Here's how the part is built. I have some questions about the finished solid (model axes, mm). A direction names the side the tool comes from. Coordinates: 2 decimals unless noted, no trailing zeros. Order: outer loops, then holes, each group sorted by start corner. A loop starts at its lowest first (then second) coordinate and runs counter-clockwise, first axis right, second up.
```python
from build123d import *

# Parameters (mm, degrees)
SKETCH1_W           = 30
SKETCH1_H           = 20
SKETCH1_R           = 1.3
BOSS_EXTRUDE1_DEPTH = 5
SKETCH2_W           = 18.5
SKETCH2_H           = 20
BOSS_EXTRUDE2_DEPTH = 70
FILLET1_R           = 1
SKETCH12_W          = 8.5
SKETCH12_H          = 10
CUT_EXTRUDE1_DEPTH  = 81
FILLET2_R           = 1


with BuildPart() as part:
    # Sketch1 → Boss-Extrude1 (new body)
    with BuildSketch(Plane(origin=(0, 0, 0), x_dir=(1, 0, 0), z_dir=(0, 1, 0))):
        Rectangle(SKETCH1_W, SKETCH1_H)
        with Locations((-12, 6)):
            Circle(SKETCH1_R, mode=Mode.SUBTRACT)
        with Locations((12, 6)):
            Circle(SKETCH1_R, mode=Mode.SUBTRACT)
        with Locations((12, -6)):
            Circle(SKETCH1_R, mode=Mode.SUBTRACT)
        with Locations((-12, -6)):
            Circle(SKETCH1_R, mode=Mode.SUBTRACT)
    boss_extrude1 = extrude(amount=BOSS_EXTRUDE1_DEPTH)

    # Sketch2 → Boss-Extrude2 (add)
    with BuildSketch(Plane(origin=(0, 5, 0), x_dir=(1, 0, 0), z_dir=(0, 1, 0))):
        Rectangle(SKETCH2_W, SKETCH2_H)
    extrude(amount=BOSS_EXTRUDE2_DEPTH)

    # Mirror1: Boss-Extrude1 across plane
    add(boss_extrude1.mirror(Plane.ZX.offset(40)))

    # Fillet1
    fillet1_edges = [part.edges().sort_by_distance(p)[0] for p in [
        (-15, 5, 0),
        (-12.125, 5, 10),
        (-12.125, 5, -10),
        (12.125, 5, 10),
        (9.25, 5, 0),
        (9.25, 40, 10),
        (9.25, 40, -10),
        (-9.25, 5, 0),
        (-9.25, 40, -10),
        (-9.25, 40, 10),
        (9.25, 75, 0),
        (-9.25, 75, 0),
        (15, 75, 0),
        (15, 77.5, -10),
        (-12.125, 75, 10),
        (12.125, 75, 10),
        (15, 77.5, 10),
        (-15, 75, 0),
        (-15, 77.5, 10),
        (12.125, 75, -10),
        (-12.125, 75, -10),
        (-15, 77.5, -10),
        (15, 5, 0),
        (15, 2.5, 10),
        (-15, 2.5, 10),
        (-15, 2.5, -10),
        (15, 2.5, -10),
        (12.125, 5, -10),
    ]]
    fillet(fillet1_edges, radius=FILLET1_R)

    # Sketch12 → Cut-Extrude1 (cut, through all)
    with BuildSketch(Plane(origin=(0, 80, 0), x_dir=(1, 0, 0), z_dir=(0, 1, 0))):
        Rectangle(SKETCH12_W, SKETCH12_H)
    extrude(amount=-CUT_EXTRUDE1_DEPTH, mode=Mode.SUBTRACT)

    # Fillet2
    fillet2_edges = [part.edges().sort_by_distance(p)[0] for p in [
        (4.25, 40, 5),
        (-4.25, 40, 5),
        (-4.25, 40, -5),
        (4.25, 40, -5),
    ]]
    fillet(fillet2_edges, radius=FILLET2_R)


solid = part.part
```
Q1. If we section it at B-B on z = -2.5: Write out the boundary of the cut face in (x, y).
Q2. If we section it at C-C on y = 16: Write out the boundary of the cut face in (x, z).
Q3. I need wall thicknesses on L1, parallel to X at y = 4, z = 6; L2, parallel to Z at x = -12, y = 79; L3, parallel to Y at x = 11.5, z = -3.5. Which ranges of each line are inside material? Lowest first, please.
Q4. If we section it at D-D on x = 12: Write out the boundary of the cut face in (y, z).
Q5. We'd pull the mould along Z, two halves only. Please class faces 1 (the flat face through (-12, 5, 0)), 2 (the flat face through (0, 41, 10)), 3 (the cylindrical face through (-11.4, 77.535, 7.153)), 4 (the flat face through (4.25, 41, 0)): pulls with the +Z half, pulls with the -Z half, needs draft (parallel to the pull), parting line crosses it, or undercut.
Q6. If we section it at A-A on x = -2.5: Write out the boundary of the cut face in (y, z).
Q7. Will these pins go through, and if not, where does the flat tip stop? pin 1 (9 mm diameter, centred on y = 41.5, z = -4, fed in from +X); pin 2 (2 mm diameter, centred on y = 52.5, z = -1, fed in from -X).
Q8. For faces 5 (the flat face through (0, 41, -5)), 6 (the flat face through (15, 78, 0)), 7 (the flat face through (12, 75, 0)), 8 (the flat face through (-12, 75, 0)), which set-ups out of +Z, -Z, +X, -X, +Y, -Y let a thin tool reach every point of the face, with its end or its side?
Reply:
1. outline: (-15, 0) - (-4.25, 0) - (-4.25, 80) - (-15, 80) - (-15, 76) arc R1 ccw to (-14, 75) - (-10.25, 75) arc R1 cw to (-9.25, 74) - (-9.25, 6) arc R1 cw to (-10.25, 5) - (-14, 5) arc R1 ccw to (-15, 4) - close; (4.25, 0) - (15, 0) - (15, 4) arc R1 ccw to (14, 5) - (10.25, 5) arc R1 cw to (9.25, 6) - (9.25, 74) arc R1 cw to (10.25, 75) - (14, 75) arc R1 ccw to (15, 76) - (15, 80) - (4.25, 80) - close
2. outline: (-9.25, -9) arc R1 ccw to (-8.25, -10) - (8.25, -10) arc R1 ccw to (9.25, -9) - (9.25, 9) arc R1 ccw to (8.25, 10) - (-8.25, 10) arc R1 ccw to (-9.25, 9) - close; hole (-4.25, -4) arc R1 ccw to (-3.25, -5) - (3.25, -5) arc R1 ccw to (4.25, -4) - (4.25, 4) arc R1 ccw to (3.25, 5) - (-3.25, 5) arc R1 ccw to (-4.25, 4) - close
3. L1: x = -15 to -13.3, -10.7 to 10.7, 13.3 to 15
3. L2: z = -10 to -7.3, -4.7 to 4.7, 7.3 to 10
3. L3: y = 0 to 5, 75 to 80
4. outline: (0, -10) - (4, -10) arc R1 ccw to (5, -9) - (5, -7.3) - (0, -7.3) - close; (0, -4.7) - (5, -4.7) - (5, 4.7) - (0, 4.7) - close; (0, 7.3) - (5, 7.3) - (5, 9) arc R1 ccw to (4, 10) - (0, 10) - close; (75, -9) arc R1 ccw to (76, -10) - (80, -10) - (80, -7.3) - (75, -7.3) - close; (75, -4.7) - (80, -4.7) - (80, 4.7) - (75, 4.7) - close; (75, 7.3) - (80, 7.3) - (80, 10) - (76, 10) arc R1 ccw to (75, 9) - close
5. face 1: needs draft
5. face 2: pulls with the +Z half
5. face 3: undercut
5. face 4: undercut
6. outline: (0, -10) - (80, -10) - (80, -5) - (0, -5) - close; (0, 5) - (80, 5) - (80, 10) - (0, 10) - close
7. pin 1: stops at x = 9.25
7. pin 2: stops at x = -9.25
8. face 5: +Y, -Y
8. face 6: +Z, -Z, +X, +Y, -Y
8. face 7: +Z, -Z, +X
8. face 8: +Z, -Z, -X
